Read the model definition and answer for the solid it produces. Units are mm, in the model's axes. Face numbers are marked on the shaded views. A direction names the side the tool comes from. Give positions to 0.01 mm unless a question says otherwise; leave off trailing zeros. Write each loop counter-clockwise with the first axis right and the second up, starting at its lowest first coordinate (ties: lowest second). Pieces come first, ordered by that corner, then holes. Notation, with made-up numbers: (5.5, 29.5) -> (61.5, 29.5) arc R14 ccw to (61.5, 42.5) -> close; hole circle Ø11 at (49.5, 2.5). An arc over 180 degrees is marked (long way). Put each result on its own line as item: value. Start each with the question number.
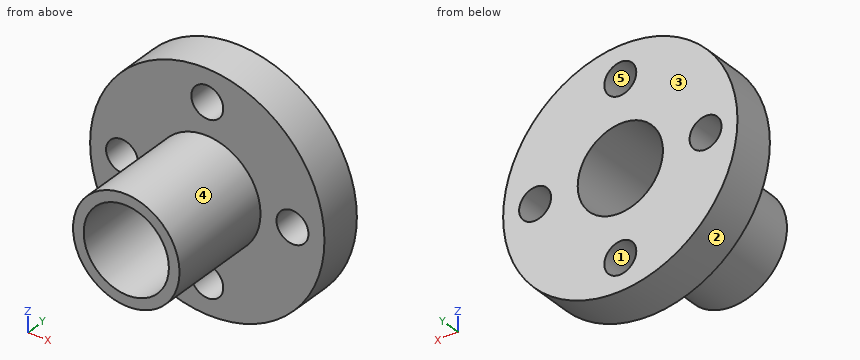
from build123d import *

# Parameters (mm, degrees)
F0_R     = 11
F1_DEPTH = 4
F2_R     = 5
F3_DEPTH = 10
F4_R     = 4
F5_DEPTH = 25
F6_R     = 1.5
F7_DEPTH = 25


with BuildPart() as f1:
    # F0 (on Front) → F1 (new body)
    with BuildSketch(Plane.XZ):
        Circle(F0_R)
    extrude(amount=F1_DEPTH)

    # F2 (on face) → F3 (join)
    with BuildSketch(Plane.XZ.offset(4)):
        Circle(F2_R)
    extrude(amount=F3_DEPTH)

    # F4 (on face) → F5 (cut)
    with BuildSketch(Plane.XZ.offset(14)):
        Circle(F4_R)
    extrude(amount=-F5_DEPTH, mode=Mode.SUBTRACT)

    # F6 (on face) → F7 (cut)
    with BuildSketch(Plane(origin=(0, 0, 0), x_dir=(-1, 0, 0), z_dir=(0, 1, 0))):
        with Locations((-8, 0)):
            Circle(F6_R)
        with Locations((0, 8)):
            Circle(F6_R)
        with Locations((8, 0)):
            Circle(F6_R)
        with Locations((0, -8)):
            Circle(F6_R)
    extrude(amount=-F7_DEPTH, mode=Mode.SUBTRACT)


solid = f1.part
1) A cutting plane is placed at B-B on z = 0. Give the vertices of the cut face in (x, y).
2) Straight lines are drawn through the part: line 1 (Z direction, x = 0, y = -1.6); line 2 (Z direction, x = -8, y = -1.8); line 3 (Y direction, x = -9, z = 2.5). For each, find the intervals that lie inside material, in ascending order. Write a range as [from, to].
3) Each of these flat-tipped pins is pushed along its axis until it touches: pin 1 Ø2 at (y, z) = (-9, 2) entering from -X; pin 2 Ø5 at (x, z) = (0, -8) entering from -Y; pin 3 Ø8 at (y, z) = (-12.5, 6.5) entering from -X. Where does it stop, or does it pass through?
4) A cutting plane is placed at A-A on x = 0. Give the vertices of the cut face in (y, z), and give its area (3 significant figures).
5) For the marked faces 4 and 5, determine the directions among +Z, -Z, +X, -X, +Y, -Y from which every point of the face is accessible in a straight line to the end or side of a thin tool.
6) For a pull along X with two mould halves and no side action, classify the marked faces 1, 2 and 3 as pulls with the +X half, pulls with the -X half, needs draft (parallel to the pull), parting line crosses it, or undercut.
7) A cutting plane is placed at D-D on x = 7.75. Give the vertices of the cut face in (y, z), and give its area (3 significant figures).
8) A cutting plane is placed at C-C on z = -8. Give the vertices of the cut face in (x, y).
Results found:
1. outline: (-11, -4) -> (-9.5, -4) -> (-9.5, 0) -> (-11, 0) -> close; (-6.5, -4) -> (-5, -4) -> (-5, -14) -> (-4, -14) -> (-4, 0) -> (-6.5, 0) -> close; (4, -14) -> (5, -14) -> (5, -4) -> (6.5, -4) -> (6.5, 0) -> (4, 0) -> close; (9.5, -4) -> (11, -4) -> (11, 0) -> (9.5, 0) -> close
2. line 1: z = [-11, -9.5], [-6.5, -4], [4, 6.5], [9.5, 11]
2. line 2: z = [-7.55, -1.5], [1.5, 7.55]
2. line 3: y = [-4, 0]
3. pin 1: stops at x = -4.9
3. pin 2: stops at y = -4
3. pin 3: stops at x = -4.33
4. outline: (-14, -5) -> (-4, -5) -> (-4, -6.5) -> (0, -6.5) -> (0, -4) -> (-14, -4) -> close; (-14, 4) -> (0, 4) -> (0, 6.5) -> (-4, 6.5) -> (-4, 5) -> (-14, 5) -> close; (-4, -11) -> (0, -11) -> (0, -9.5) -> (-4, -9.5) -> close; (-4, 9.5) -> (0, 9.5) -> (0, 11) -> (-4, 11) -> close
4. area: 52.0 mm²
5. face 4: -Y
5. face 5: +Y, -Y
6. face 1: undercut
6. face 2: parting line crosses it
6. face 3: needs draft
7. outline: (-4, -7.81) -> (0, -7.81) -> (0, -1.48) -> (-4, -1.48) -> close; (-4, 1.48) -> (0, 1.48) -> (0, 7.81) -> (-4, 7.81) -> close
7. area: 50.6 mm²
8. outline: (-7.55, -4) -> (-1.5, -4) -> (-1.5, 0) -> (-7.55, 0) -> close; (1.5, -4) -> (7.55, -4) -> (7.55, 0) -> (1.5, 0) -> close
